Read the model definition and answer for the solid it produces. Units are mm, in the model's axes. A direction names the side the tool comes from. Round coordinates to 2 decimals unless told otherwise and drop trailing zeros. Write each loop counter-clockwise with the first axis right and the second up, starting at its lowest first coordinate (ties: lowest second). Pieces come first, ordered by that corner, then holes. Notation, with made-up numbers: (7, -10) - (59, -10) arc R27 cw to (59, 29) - close; hole circle Ø9 at (9.5, 14.5). An arc over 180 degrees is marked (long way). Use one line per item in the form item = value. Start each with the question number.
1) The part is cut by section C-C, the plane y = -105.5. Count the separate pieces of the cut face and the enclosed holes in it, plus the area to 3 significant figures.
2) Consider line 1 along Z through (x, y) = (234, -34); line 2 along X through (y, z) = (-25, 328). Determine where each line is inside the solid, lowest interval first. Write a range as from..to.
3) The part is cut by section B-B, the plane x = 1086. Give the vertices of the cut face in (y, z), plus the area to 3 significant figures.
4) For faces 1 (the face through (1850, -197, 690)), 2 (the face through (1400, -197, 247)), determine the directions among +Z, -Z, +X, -X, +Y, -Y from which every point of the face is accessible in a straight line to the end or side of a thin tool.
5) This flat-tipped pin is pushed along its axis until it touches: pin 1 (9 mm diameter, centred on x = 808, z = -9.5, fed in from -Y). Where does it stop, or does it pass through?
6) For a pull along Z with two mould halves and no side action, classify faces 3 (the face through (921, -400, 548)), 4 (the face through (450, -197, 247)) as released by +Z, released by -Z, zero draft, split by the parting line, or undercut.
7) The part is cut by section A-A, the plane z = 1030. Give the vertices of the cut face in (x, y), plus the area to 3 significant figures.
from build123d import *

# Parameters (mm, degrees)
F0_W     = 1850
F0_H     = 1400
F0_W_2   = 400
F0_H_2   = 400
F1_DEPTH = 400
F2_W     = 1810
F2_H     = 360
F3_DEPTH = 30


with BuildPart() as f1:
    # F0 (on Front) → F1 (new body)
    with BuildSketch(Plane.XZ):
        with Locations((925, 700)):
            Rectangle(F0_W, F0_H)
        with Locations((250, 250)):
            Rectangle(F0_W_2, F0_H_2, mode=Mode.SUBTRACT)
        with Locations((700, 250)):
            Rectangle(F0_W_2, F0_H_2, mode=Mode.SUBTRACT)
        with Locations((1150, 250)):
            Rectangle(F0_W_2, F0_H_2, mode=Mode.SUBTRACT)
        with Locations((1600, 250)):
            Rectangle(F0_W_2, F0_H_2, mode=Mode.SUBTRACT)
        with Locations((250, 700)):
            Rectangle(F0_W_2, F0_H_2, mode=Mode.SUBTRACT)
        with Locations((700, 700)):
            Rectangle(F0_W_2, F0_H_2, mode=Mode.SUBTRACT)
        with Locations((250, 1150)):
            Rectangle(F0_W_2, F0_H_2, mode=Mode.SUBTRACT)
        with Locations((700, 1150)):
            Rectangle(F0_W_2, F0_H_2, mode=Mode.SUBTRACT)
        with Locations((1150, 700)):
            Rectangle(F0_W_2, F0_H_2, mode=Mode.SUBTRACT)
        with Locations((1600, 700)):
            Rectangle(F0_W_2, F0_H_2, mode=Mode.SUBTRACT)
        with Locations((1150, 1150)):
            Rectangle(F0_W_2, F0_H_2, mode=Mode.SUBTRACT)
        with Locations((1600, 1150)):
            Rectangle(F0_W_2, F0_H_2, mode=Mode.SUBTRACT)
    extrude(amount=F1_DEPTH)

    # F2 (on face) → F3 (join)
    with BuildSketch(Plane(origin=(0, 0, 0), x_dir=(1, 0, 0), z_dir=(0, 0, -1))):
        with Locations((925, 200)):
            Rectangle(F2_W, F2_H)
    extrude(amount=F3_DEPTH)


solid = f1.part
Geometry results:
q1.separate_pieces = 1
q1.enclosed_holes = 12
q1.area = 724,000 mm2
q2.line_1 = -30..50, 450..500, 900..950, 1350..1400
q2.line_2 = 0..50, 450..500, 900..950, 1350..1400, 1800..1850
q3.outline = (-400, 0) - (-380, 0) - (-380, -30) - (-20, -30) - (-20, 0) - (0, 0) - (0, 50) - (-400, 50) - close; (-400, 450) - (0, 450) - (0, 500) - (-400, 500) - close; (-400, 900) - (0, 900) - (0, 950) - (-400, 950) - close; (-400, 1350) - (0, 1350) - (0, 1400) - (-400, 1400) - close
q3.area = 90,800 mm2
q4.face_1 = +Z, -Z, +X, +Y, -Y
q4.face_2 = +Y, -Y
q5.pin_1 = -380
q6.face_3 = zero draft
q6.face_4 = undercut
q7.outline = (0, -400) - (50, -400) - (50, 0) - (0, 0) - close; (450, -400) - (500, -400) - (500, 0) - (450, 0) - close; (900, -400) - (950, -400) - (950, 0) - (900, 0) - close; (1350, -400) - (1400, -400) - (1400, 0) - (1350, 0) - close; (1800, -400) - (1850, -400) - (1850, 0) - (1800, 0) - close
q7.area = 100,000 mm2
